from build123d import *

# Parameters (mm, degrees)
F0_W           = 35
F0_H           = 35
F1_DEPTH       = 9
F2_R           = 14
F2_R_2         = 13
F3_DEPTH       = 14
F4_DEPTH       = 9.001
F6_D           = 3.4
F6_CBORE_D     = 6.5
F6_CBORE_DEPTH = 4
F7_DEPTH       = 23.001
F8_R           = 14
F8_R_2         = 12
F9_DEPTH       = 9
F10_SIZE       = 0.5


with BuildPart() as f1:
    # F0 (on Top) → F1 (new body)
    with BuildSketch(Plane.XY):
        Rectangle(F0_W, F0_H)
    extrude(amount=F1_DEPTH)

    # F2 (on face) → F3 (join)
    with BuildSketch(Plane(origin=(0, 0, 0), x_dir=(1, 0, 0), z_dir=(0, 0, -1))):
        Circle(F2_R)
        Circle(F2_R_2, mode=Mode.SUBTRACT)
    extrude(amount=F3_DEPTH)

    # F4 (cut, through all): a face of the model
    f4_faces = [f1.faces().sort_by_distance(p)[0] for p in [
        (0, 0, 0),
    ]]
    extrude(f4_faces, amount=-F4_DEPTH, mode=Mode.SUBTRACT)

    # F6 (through all)
    with Locations(Plane.XY.offset(9)):
        with Locations((-12.3743686708, 12.3743686708), (12.3743686708, 12.3743686708), (-12.3743686708, -12.3743686708), (12.3743686708, -12.3743686708)):
            CounterBoreHole(F6_D / 2, F6_CBORE_D / 2, F6_CBORE_DEPTH)

    # F5 (on face) → F7 (cut, through all)
    with BuildSketch(Plane.XY.offset(9)):
        with BuildLine():
            ThreePointArc((12.4899959968, 17.5), (15.2027957955, 15.2027957955), (17.5, 12.4899959968))
            Line((17.5, 12.4899959968), (17.5, 17.5))
            Line((17.5, 17.5), (12.4899959968, 17.5))
        make_face()
        with BuildLine():
            ThreePointArc((-17.5, 12.4899959968), (-15.2027957955, 15.2027957955), (-12.4899959968, 17.5))
            Line((-12.4899959968, 17.5), (-17.5, 17.5))
            Line((-17.5, 17.5), (-17.5, 12.4899959968))
        make_face()
        with BuildLine():
            Line((-17.5, -17.5), (-12.4899959968, -17.5))
            ThreePointArc((-12.4899959968, -17.5), (-15.2027957955, -15.2027957955), (-17.5, -12.4899959968))
            Line((-17.5, -12.4899959968), (-17.5, -17.5))
        make_face()
        with BuildLine():
            Line((17.5, -17.5), (17.5, -12.4899959968))
            ThreePointArc((17.5, -12.4899959968), (15.2027957955, -15.2027957955), (12.4899959968, -17.5))
            Line((12.4899959968, -17.5), (17.5, -17.5))
        make_face()
    extrude(amount=-F7_DEPTH, mode=Mode.SUBTRACT)

    # F8 (on face) → F9 (join)
    with BuildSketch(Plane(origin=(0, 0, 0), x_dir=(1, 0, 0), z_dir=(0, 0, -1))):
        Circle(F8_R)
        Circle(F8_R_2, mode=Mode.SUBTRACT)
    extrude(amount=-F9_DEPTH)

    # F10
    f10_edges = [f1.edges().sort_by_distance(p)[0] for p in [
        (0, -17.5, 9),
        (-15.202796, -15.202796, 9),
        (0, 17.5, 9),
        (15.202796, 15.202796, 9),
        (17.5, 0, 9),
        (-15.202796, 15.202796, 9),
        (15.202796, -15.202796, 9),
        (-17.5, 0, 9),
    ]]
    chamfer(f10_edges, length=F10_SIZE)


solid = f1.part
Can you work these out from the model? Positions are in its coordinate system, mm. A direction names the side the tool comes from. Coordinates: 2 decimals unless noted, no trailing zeros. Write each loop counter-clockwise with the first axis right and the second up, starting at its lowest first coordinate (ties: lowest second). Pieces come first, ordered by that corner, then holes.
Q1. Please list where these lines run through material, in increasing order: L1, parallel to Y at x = 0, z = -9; L2, parallel to X at y = 14, z = 5.5.
Results found:
L1: y = -14 to -13, 13 to 14
L2: x = -16.32 to -15.19, -9.56 to 9.56, 15.19 to 16.32
Q2. Which directions (+Z, -Z, +X, -X, +Y, -Y) give clear straight access to the entire face, cutting with the end or side of a thin tool? Please do faces 1 (the face through (0, 17.5, 4)), 2 (the face through (-10.627, 15.115, 7.028)), 3 (the face through (9, 9, 0)).
Results found:
face 1: +Z, -Z, +X, -X, +Y
face 2: +Z
face 3: -Z
Q3. Imagine slicing it at A-A, the plane x = 0. List the corners of the cut face in (y, z) for me, plus the area to 3 significant figures.
Results found:
outline: (-17.5, 0) - (-14, 0) - (-14, -14) - (-13, -14) - (-13, 0) - (-12, 0) - (-12, 9) - (-17, 9) - (-17.5, 8.5) - close; (12, 0) - (13, 0) - (13, -14) - (14, -14) - (14, 0) - (17.5, 0) - (17.5, 8.5) - (17, 9) - (12, 9) - close
area: 127 mm2
Q4. Imagine slicing it at D-D, the plane z = -3.5. List the corners of the cut face in (x, y) for me.
Results found:
outline: circle Ø28 at (0, 0); hole circle Ø26 at (0, 0)
Q5. If we mould it in two halves opening along Y, with no side actions, what happens to faces 4 (the face through (-15.238, 15.168, 4.31)), 5 (the face through (-13.079, -15.547, 7.028)), 6 (the face through (15.238, -15.168, 4.31)), 7 (the face through (12.932, 5.362, -6.902))? For each: +Y half, -Y half, draft (parallel to the pull), parting line (faces both ways), or undercut.
Results found:
face 4: +Y half
face 5: undercut
face 6: -Y half
face 7: parting line
Q6. For P1, Ø6, axis at x = 12.37, y = 12.37, coming from the -Z side; P2, Ø4, axis at x = -12.37, y = -12.37, coming from the +Z side; P3, Ø10, axis at x = 12, z = -8, coming from the +Y side, each with a flat end and sliding along its axis, tell me the tip position at first contact or that it passes through.
Results found:
P1: stops at z = 0
P2: stops at z = 5
P3: stops at y = 12.12
Q7. Imagine slicing it at C-C, the plane z = 3.5. List the corners of the cut face in (x, y) for me, plus the area to 3 significant figures.
Results found:
outline: (-17.5, -12.49) arc R21.5 ccw to (-12.49, -17.5) - (12.49, -17.5) arc R21.5 ccw to (17.5, -12.49) - (17.5, 12.49) arc R21.5 ccw to (12.49, 17.5) - (-12.49, 17.5) arc R21.5 ccw to (-17.5, 12.49) - close; hole circle Ø3.4 at (-12.37, -12.37); hole circle Ø3.4 at (-12.37, 12.37); hole circle Ø24 at (0, 0); hole circle Ø3.4 at (12.37, -12.37); hole circle Ø3.4 at (12.37, 12.37)
area: 692 mm2
